Design review of the part built by this model. Coordinates are the model's own, in mm. A direction names the side the tool comes from. Give positions to 0.01 mm unless a question says otherwise; leave off trailing zeros. Write each loop counter-clockwise with the first axis right and the second up, starting at its lowest first coordinate (ties: lowest second). Pieces come first, ordered by that corner, then holes. Notation, with made-up numbers: (-33, 1) -> (9, 1) arc R32 cw to (9, 31) -> close; hole circle Ø4 at (-17.5, -23). An arc over 180 degrees is marked (long way). Return JSON: item names as keys, results as strings. Group by question number.
from build123d import *

# Parameters (mm, degrees)
F0_W     = 61
F0_H     = 49
F1_DEPTH = 1.7
F3_W     = 11
F3_H     = 7
F4_DEPTH = 1
F5_R     = 8
F6_DEPTH = 8
F7_R     = 6.2
F8_DEPTH = 3


with BuildPart() as f1:
    # F0 (on Top) → F1 (new body)
    with BuildSketch(Plane.XY):
        with Locations((-30.5, 24.5)):
            Rectangle(F0_W, F0_H)
    extrude(amount=F1_DEPTH)

    # F3 (on offset) → F4 (join)
    with BuildSketch(Plane.YZ.offset(-8)):
        Polygon((4, 8.7), (19, 8.7), (30, 8.7), (45, 8.7), (45, 37.2), (4, 37.2), align=None)
        with Locations((24.5, 5.2)):
            Rectangle(F3_W, F3_H)
    extrude(amount=-F4_DEPTH)

    # F5 (on face) → F6 (join)
    with BuildSketch(Plane.YZ.offset(-8)):
        with Locations((24.5, 22.2)):
            Circle(F5_R)
    extrude(amount=F6_DEPTH)

    # F7 (on face) → F8 (join)
    with BuildSketch(Plane.YZ):
        with Locations((24.5, 22.2)):
            Circle(F7_R)
    extrude(amount=F8_DEPTH)


solid = f1.part
Q1. Take a section at C-C, the plane z = 22.2. Give the boundary of the cut face in (x, y), plus the area to 3 significant figures.
Q2. For L1, parallel to X at y = 8.5, z = 18.5; L2, parallel to Z at x = -50, y = 12.5; L3, parallel to X at y = 31.5, z = 20, list the stretches that pass through material, from the lowest coordinate up. Write a range as from..to.
Q3. Take a section at D-D, the plane y = 24.5. Give the boundary of the cut face in (x, z).
Q4. Take a section at A-A, the plane y = 42. Give the boundary of the cut face in (x, z), plus the area to 3 significant figures.
Q5. Take a section at B-B, the plane x = -1.5. Give the boundary of the cut face in (y, z).
Q6. Insertion check: pin 1 (5 mm diameter, centred on x = -44.5, y = 30, fed in from +Z); pin 2 (0.8 mm diameter, centred on y = 15, z = 0.5, fed in from +X); pin 3 (0.5 mm diameter, centred on x = -8.5, z = 4, fed in from +Y). Each pin has a flat end and moves straight along its axis. Give the tip position at first contact, or say it passes through.
Q7. Tool access review of faces 1 (the face through (0, 24, 1)), 2 (the face through (-9, 24, 24)), 3 (the face through (-31, 49, 1)), 4 (the face through (-61, 24, 1)), 5 (the face through (-4.06, 22.77, 14.39)): name each direction out of +Z, -Z, +X, -X, +Y, -Y from which nothing blocks a thin tool from reaching the whole face with its end or side.
Final values:
{
 "1": {"outline": "(-9, 4) -> (-8, 4) -> (-8, 16.5) -> (0, 16.5) -> (0, 18.3) -> (3, 18.3) -> (3, 30.7) -> (0, 30.7) -> (0, 32.5) -> (-8, 32.5) -> (-8, 45) -> (-9, 45) -> close", "area": "206 mm²"},
 "2": {"L1": "x = -9..-8", "L2": "z = 0..1.7", "L3": "x = -9..0"},
 "3": {"outline": "(-61, 0) -> (0, 0) -> (0, 1.7) -> (-8, 1.7) -> (-8, 14.2) -> (0, 14.2) -> (0, 16) -> (3, 16) -> (3, 28.4) -> (0, 28.4) -> (0, 30.2) -> (-8, 30.2) -> (-8, 37.2) -> (-9, 37.2) -> (-9, 1.7) -> (-61, 1.7) -> close"},
 "4": {"outline": "(-61, 0) -> (0, 0) -> (0, 1.7) -> (-61, 1.7) -> close; (-9, 8.7) -> (-8, 8.7) -> (-8, 37.2) -> (-9, 37.2) -> close", "area": "132 mm²"},
 "5": {"outline": "(0, 0) -> (49, 0) -> (49, 1.7) -> (0, 1.7) -> close; circle Ø16 at (24.5, 22.2)"},
 "6": {"pin 1": "stops at z = 1.7", "pin 2": "stops at x = 0", "pin 3": "stops at y = 30"},
 "7": {"face 1": "-Z, +X, +Y, -Y", "face 2": "+Z, -X, +Y, -Y", "face 3": "+Z, -Z, +X, -X, +Y", "face 4": "+Z, -Z, -X, +Y, -Y", "face 5": "+X"}
}
